Can you work these out from the model? Positions are in its coordinate system, mm. A direction names the side the tool comes from. Give positions to 0.01 mm unless a question says otherwise; leave off trailing zeros. Loops run counter-clockwise (first coordinate to the right, second up) from the corner with the lowest first, then second, coordinate; pieces in that order, holes last.
Autodesk Fusion 360 part; units mm, degrees
sketch "Top" plane through (0, 0, 0) normal (0, 0, 1) x (1, 0, 0)
  line L0 (0, 0) -> (40, 0)
  line L1 (40, 0) -> (40, 50)
  line L2 (40, 50) -> (0, 50)
  line L3 (0, 50) -> (0, 0)
  circle A0 centre (20, 25) radius 11.2
  circle A1 centre (20, 25) radius 6
  dimension "d6" = 40
  dimension "d7" = 50
  dimension "d11" = 22.4
  dimension "d12" = 25
  dimension "d13" = 20
  dimension "d27" = 12
extrude "Extrude1" add sketch "Top" along normal blind 10 contours L0 L1 L2 L3 | A0 | A1
extrude "Extrude2" cut sketch "Top" along normal blind 8 contours A0 | A1
extrude "Extrude5" cut sketch "Top" along normal blind 110 contours A1
sketch "Sketch5" plane through (0, 0, 0) normal (-1, 0, 0) x (0, -1, 0)
  line L0 (-50, 0) -> (0, 0)
  line L1 (0, 0) -> (0, 10)
  line L2 (0, 10) -> (-50, 10)
  line L3 (-50, 10) -> (-50, 0)
  line L4 (-48, 10) -> (-38, 10)
  line L5 (-38, 10) -> (-38, 0)
  line L6 (-38, 0) -> (-48, 0)
  line L7 (-48, 0) -> (-48, 10)
  dimension "d50" = 10
  dimension "d51" = 10
  dimension "d52" = 2
extrude "Extrude8" add sketch "Sketch5" along normal blind 30 contours L0 L2 L4 L5 L6 L7
sketch "Sketch8" plane through (40, 0, 0) normal (1, 0, 0) x (0, 1, 0)
  line L0 (0, 0) -> (50, 0)
  line L1 (50, 0) -> (50, 10)
  line L2 (50, 10) -> (0, 10)
  line L3 (0, 10) -> (0, 0)
  line L4 (2, 10) -> (12, 10)
  line L5 (12, 10) -> (12, 0)
  line L6 (12, 0) -> (2, 0)
  line L7 (2, 0) -> (2, 10)
  dimension "d72" = 10
  dimension "d73" = 10
  dimension "d74" = 2
extrude "Extrude11" add sketch "Sketch8" along normal blind 30 contours L0 L2 L4 L5 L6 L7
sketch "Sketch9" plane through (0, 0, 0) normal (0, 0, -1) x (1, 0, 0)
  circle A0 centre (20, -25) radius 11.2
  line L0 (0, -48) -> (0, -50)
  line L1 (0, -50) -> (40, -50)
  line L2 (40, -50) -> (40, -12)
  line L3 (40, -12) -> (70, -12)
  line L4 (70, -12) -> (70, -2)
  line L5 (70, -2) -> (40, -2)
  line L6 (40, -2) -> (40, 0)
  line L7 (40, 0) -> (0, 0)
  line L8 (0, 0) -> (0, -38)
  line L9 (0, -38) -> (-30, -38)
  line L10 (-30, -38) -> (-30, -48)
  line L11 (-30, -48) -> (0, -48)
  circle A1 centre (-27.2, -43) radius 0.8
  circle A2 centre (67.2, -7) radius 0.8
  dimension "d81" = 1.6
  dimension "d82" = 1.6
  dimension "d83" = 2.8
  dimension "d84" = 5
  dimension "d85" = 2.8
  dimension "d86" = 5
extrude "Extrude12" add sketch "Sketch9" along normal blind 10 contours A1 | A2
equation "length = 50 mm"
equation "width = 40 mm"
equation "thickness = 10 mm"
equation "extra = 100 mm"
equation "fit_gap = 0.2 mm"
equation "d6 = width"
equation "d7 = length"
equation "d8 = thickness"
equation "bearing_outer_radius = 11.1 mm"
equation "d11 = ( bearing_outer_radius * 2 ) + fit_gap"
equation "d12 = length / 2"
equation "d13 = width / 2"
equation "d14 = thickness - 2 mm"
equation "bearing_inner_radius = ( 8 mm + 4 mm ) / 2"
equation "d27 = bearing_inner_radius * 2"
equation "d28 = thickness + extra"
equation "rack_rock_bracket_length = 30 mm"
equation "rack_rock_bracket_width = 10 mm"
equation "rack_rock_bracket_big_distance = 2 mm"
equation "d50 = rack_rock_bracket_width"
equation "d51 = rack_rock_bracket_width"
equation "d52 = rack_rock_bracket_big_distance"
equation "d53 = rack_rock_bracket_length"
equation "d72 = rack_rock_bracket_width"
equation "d73 = rack_rock_bracket_width"
equation "d74 = rack_rock_bracket_big_distance"
equation "d75 = rack_rock_bracket_length"
equation "bearing_dowel_radius = 0.8 mm"
equation "bearing_dowel_length = 10 mm"
equation "bearing_dowel_big_distance = 2 mm + bearing_dowel_radius"
equation "bearing_dowel_small_distance = rack_rock_bracket_width / 2"
equation "d81 = bearing_dowel_radius * 2"
equation "d82 = bearing_dowel_radius * 2"
equation "d83 = bearing_dowel_big_distance"
equation "d84 = bearing_dowel_small_distance"
equation "d85 = bearing_dowel_big_distance"
equation "d86 = bearing_dowel_small_distance"
equation "d87 = bearing_dowel_length"
(1) Please list where these lines run through material, in increasing order: probe 1 along Y at (x, z) = (20, 5); probe 2 along Y at (x, z) = (20, 9); probe 3 along X at (y, z) = (25, 8.7).
Returned:
probe 1: y = 0 to 13.8, 36.2 to 50
probe 2: y = 0 to 19, 31 to 50
probe 3: x = 0 to 14, 26 to 40
(2) Thinking about a two-plate mould opening in Y: for faces 6 (the cylindrical face through (25.54, 27.3, 8.99)), 7 (the cylindrical face through (17.572, 35.934, 3.944)), 8 (the flat face through (-15, 48, 5)), 9 (the flat face through (55, 2, 5)), which applies, pulls with the +Y half, pulls with the -Y half, needs draft (parallel to the pull), parting line crosses it, or undercut?
Returned:
face 6: undercut
face 7: undercut
face 8: pulls with the +Y half
face 9: pulls with the -Y half
(3) Which directions (+Z, -Z, +X, -X, +Y, -Y) give clear straight access to the entire face, cutting with the end or side of a thin tool? Please do faces 1 (the flat face through (40, 1, 5)), 2 (the flat face through (0, 19, 5)), 3 (the flat face through (0, 49, 5)), 4 (the flat face through (25, 20, 8)), 5 (the flat face through (55, 12, 5)).
Returned:
face 1: +Z, -Z, +X, -Y
face 2: +Z, -Z, -X, -Y
face 3: +Z, -Z, -X, +Y
face 4: -Z
face 5: +Z, -Z, +X, +Y
(4) Suppose I cut it at D-D on x = -4.5. List the corners of the cut face in (y, z) for me.
Returned:
outline: (38, 0) - (48, 0) - (48, 10) - (38, 10) - close
(5) Suppose I cut it at B-B on y = 25. List the corners of the cut face in (x, z) for me.
Returned:
outline: (0, 0) - (8.8, 0) - (8.8, 8) - (14, 8) - (14, 10) - (0, 10) - close; (26, 8) - (31.2, 8) - (31.2, 0) - (40, 0) - (40, 10) - (26, 10) - close
(6) Will these pins go through, and if not, where does the flat tip stop? P1, Ø12, axis at y = 27.5, z = 6, coming from the -X side; P2, Ø11, axis at x = -21.5, z = 5, coming from the -Y side; P3, Ø11, axis at x = 19.5, y = 30, coming from the -Z side; P4, Ø5, axis at x = -4.5, y = 8, coming from the -Z side.
Returned:
P1: stops at x = 0
P2: stops at y = 38
P3: stops at z = 8
P4: passes through
(7) Suppose I cut it at A-A on x = 20. List the corners of the cut face in (y, z) for me.
Returned:
outline: (0, 0) - (13.8, 0) - (13.8, 8) - (19, 8) - (19, 10) - (0, 10) - close; (31, 8) - (36.2, 8) - (36.2, 0) - (50, 0) - (50, 10) - (31, 10) - close
(8) Suppose I cut it at C-C on z = 1.5. List the corners of the cut face in (x, y) for me.
Returned:
outline: (-30, 38) - (0, 38) - (0, 0) - (40, 0) - (40, 2) - (70, 2) - (70, 12) - (40, 12) - (40, 50) - (0, 50) - (0, 48) - (-30, 48) - close; hole circle Ø22.4 at (20, 25)
